```python
from build123d import *

# Parameters (mm, degrees)
SKETCH_W   = 12
SKETCH_H   = 28
SKETCH_R   = 0.5
SKETCH_R_2 = 2
PAD_DEPTH  = 1
BOX_W      = 12
BOX_H      = 16
BOX_DEPTH  = 10


with BuildPart() as pad:
    # Sketch → Pad (new body)
    with BuildSketch(Plane.XY):
        with Locations((0, 0.964269)):
            Rectangle(SKETCH_W, SKETCH_H)
        with Locations((0, -12.035731)):
            Circle(SKETCH_R, mode=Mode.SUBTRACT)
        with Locations((2.5, -12.035731)):
            Circle(SKETCH_R, mode=Mode.SUBTRACT)
        with Locations((-2.5, -12.035731)):
            Circle(SKETCH_R, mode=Mode.SUBTRACT)
        with Locations((0, -7.035731)):
            Circle(SKETCH_R_2, mode=Mode.SUBTRACT)
    extrude(amount=PAD_DEPTH)


with BuildPart() as fusion:
    # Box → Box (new body)
    with BuildSketch(Plane(origin=(-6, -1, 0), x_dir=(1, 0, 0), z_dir=(0, 0, 1))):
        with Locations((6, 8)):
            Rectangle(BOX_W, BOX_H)
    extrude(amount=BOX_DEPTH)

    # Fusion: union Pad
    add(pad.part)


solid = fusion.part
```
Work out the finished part from the listing and answer in its coordinate system (mm). A direction names the side the tool comes from. Give positions to 0.01 mm unless a question says otherwise; leave off trailing zeros. Order: outer loops, then holes, each group sorted by start corner. A loop starts at its lowest first (then second) coordinate and runs counter-clockwise, first axis right, second up.
1. Straight lines are drawn through the part: L1, parallel to Y at x = 0, z = 0.6; L2, parallel to Y at x = 2.5, z = 0.85; L3, parallel to Z at x = -1.25, y = -4. For each, find the intervals that lie inside material, in ascending order.
Result sheet:
L1: y = -13.04 to -12.54, -11.54 to -9.04, -5.04 to 15
L2: y = -13.04 to -12.54, -11.54 to 15
L3: z = 0 to 1
2. This flat-tipped pin is pushed along its axis until it touches: P1, Ø6, axis at x = -3, y = 0, coming from the -Z side. Where does it stop, or does it pass through?
Result sheet:
P1: stops at z = 0
3. The mould has two halves that part along X. Classify faces 1 (the flat face through (6, 7, 5)), 2 (the flat face through (0, -4, 1)), 3 (the cylindrical face through (-0.07, -11.54, 0.49)): released by +X, released by -X, zero draft, split by the parting line, or undercut.
Result sheet:
face 1: released by +X
face 2: zero draft
face 3: undercut
4. Section C-C, the plane y = -11 is taken. Determine the outline of the cut face in (x, z), and give its area (3 significant figures).
Result sheet:
outline: (-6, 0) - (6, 0) - (6, 1) - (-6, 1) - close
area: 12.0 mm2
5. For faces 4 (the flat face through (0, -1, 5)), 5 (the flat face through (0, 7, 10)), determine the directions among +Z, -Z, +X, -X, +Y, -Y from which every point of the face is accessible in a straight line to the end or side of a thin tool.
Result sheet:
face 4: +Z, +X, -X, -Y
face 5: +Z, +X, -X, +Y, -Y
6. Section B-B, the plane x = -2.5 is taken. Determine the outline of the cut face in (y, z).
Result sheet:
outline: (-13.04, 0) - (-12.54, 0) - (-12.54, 1) - (-13.04, 1) - close; (-11.54, 0) - (15, 0) - (15, 10) - (-1, 10) - (-1, 1) - (-11.54, 1) - close
7. Section D-D, the plane z = 6.5 is taken. Determine the outline of the cut face in (x, y), and give its area (3 significant figures).
Result sheet:
outline: (-6, -1) - (6, -1) - (6, 15) - (-6, 15) - close
area: 192 mm2
8. Section A-A, the plane x = 0 is taken. Determine the outline of the cut face in (y, z).
Result sheet:
outline: (-13.04, 0) - (-12.54, 0) - (-12.54, 1) - (-13.04, 1) - close; (-11.54, 0) - (-9.04, 0) - (-9.04, 1) - (-11.54, 1) - close; (-5.04, 0) - (15, 0) - (15, 10) - (-1, 10) - (-1, 1) - (-5.04, 1) - close
